from build123d import *

# Parameters (mm, degrees)
PAD031_DEPTH    = 50.8
SKETCH066_R     = 2.286
POCKET030_DEPTH = 5.08
SKETCH070_R     = 2.286
POCKET033_DEPTH = 4.318


with BuildPart() as part:
    # Sketch065 → Pad031 (new body)
    with BuildSketch(Plane.YZ):
        Polygon((0, 0), (0, 33.02), (44.45, 0), align=None)
    extrude(amount=PAD031_DEPTH)

    # Sketch066 (on Face1 of Pad031) → Pocket030 (cut)
    with BuildSketch(Plane(origin=(0, 0, 0), x_dir=(0, 0, -1), z_dir=(0, -1, 0))):
        with Locations((-24.638, 18.415)):
            Circle(SKETCH066_R)
        with Locations((-18.288, 37.465)):
            Circle(SKETCH066_R)
    extrude(amount=-POCKET030_DEPTH, mode=Mode.SUBTRACT)

    # Sketch070 (on Face5 of Pocket030) → Pocket033 (cut)
    with BuildSketch(Plane(origin=(0, 15.8065228827, 21.2780115729), x_dir=(0, -0.802743848, 0.5963240013), z_dir=(0, 0.5963240013, 0.802743848))):
        with Locations((-24.7593814758, 38.1)):
            Circle(SKETCH070_R)
        with Locations((13.3406185242, 38.1)):
            Circle(SKETCH070_R)
        with Locations((13.3406185242, 12.7)):
            Circle(SKETCH070_R)
        with Locations((-24.7593814758, 12.7)):
            Circle(SKETCH070_R)
    extrude(amount=-POCKET033_DEPTH, mode=Mode.SUBTRACT)


with BuildPart() as part_1:
    # Body023 placement: moved
    add(part.part.moved(Location((-66.04, 63.5, -3.048))))


solid = part_1.part
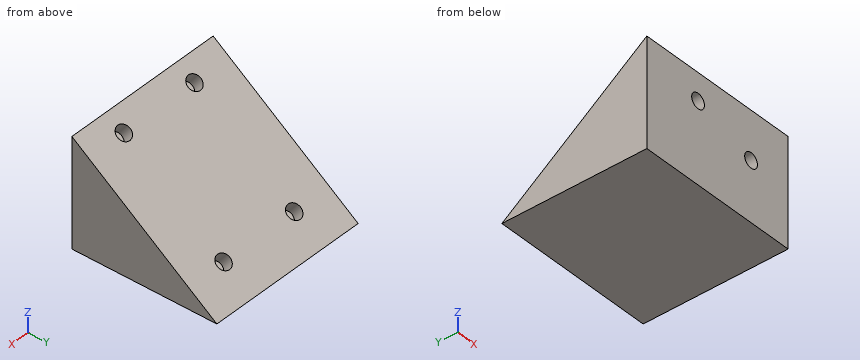
Design review of the part built by this model. Coordinates are the model's own, in mm. Coordinates: 2 decimals unless noted, no trailing zeros. Write each loop counter-clockwise with the first axis right and the second up, starting at its lowest first coordinate (ties: lowest second). Pieces come first, ordered by that corner, then holes. Notation, with made-up numbers: (58.5, 55) - (96.5, 55) arc R12 ccw to (96.5, 67) - close; hole circle Ø8 at (47.5, 42.25). An arc over 180 degrees is marked (long way). One line per item, written item: value.
1) Add section C-C (y = 79). State the section outline as (x, z) points.
Answer sheet:
outline: (-66.04, -3.05) - (-15.24, -3.05) - (-15.24, 18.46) - (-66.04, 18.46) - close
2) Add section B-B (x = -27). State the section outline as (y, z) points.
Answer sheet:
outline: (63.5, -3.05) - (107.95, -3.05) - (100.85, 2.22) - (98.28, -1.24) - (94.93, 1.24) - (97.51, 4.71) - (70.27, 24.94) - (67.7, 21.48) - (64.35, 23.96) - (66.92, 27.43) - (63.5, 29.97) - (63.5, 16.9) - (68.58, 16.9) - (68.58, 13.58) - (63.5, 13.58) - close
3) Insertion check: pin 1 (4 mm diameter, centred on x = -41.5, y = 92, fed in from +Z); pin 2 (5.5 mm diameter, centred on x = -47.625, z = 21.59, fed in from +Y); pin 3 (2.5 mm diameter, centred on x = -28.575, z = 15.24, fed in from +Y). Each pin has a flat end and moves straight along its axis. Give the tip position at first contact, or say it passes through.
Answer sheet:
pin 1: stops at z = 10.29
pin 2: stops at y = 78.49
pin 3: stops at y = 85.01
4) To check wall thickness, follow probe 1 along X at (y, z) = (64.75, 21.59); probe 2 along X at (y, z) = (67.1, 15.24); probe 3 along Z at (x, y) = (-46.5, 68). State the ranges of each line that lie inside material, in increasing order.
Answer sheet:
probe 1: x = -66.04 to -49.91, -45.34 to -15.24
probe 2: x = -66.04 to -30.86, -26.29 to -15.24
probe 3: z = -3.05 to 19.6, 23.58 to 26.63
5) Add section D-D (x = -55). State the section outline as (y, z) points, plus the area to 3 significant figures.
Answer sheet:
outline: (63.5, -3.05) - (107.95, -3.05) - (100.44, 2.53) - (97.87, -0.94) - (95.35, 0.94) - (97.92, 4.4) - (69.86, 25.25) - (67.28, 21.78) - (64.76, 23.66) - (67.34, 27.12) - (63.5, 29.97) - close
area: 707 mm2
6) Add section A-A (z = 16.5). State the section outline as (x, y) points, plus the area to 3 significant figures.
Answer sheet:
outline: (-66.04, 63.5) - (-30.48, 63.5) - (-30.48, 68.58) - (-26.67, 68.58) - (-26.67, 63.5) - (-15.24, 63.5) - (-15.24, 81.64) - (-66.04, 81.64) - close
area: 902 mm2
